Geometry check sheet. Reference: the model listing, model coordinates, mm. A direction names the side the tool comes from. Round coordinates to 2 decimals unless told otherwise and drop trailing zeros. Write each loop counter-clockwise with the first axis right and the second up, starting at its lowest first coordinate (ties: lowest second). Pieces come first, ordered by that corner, then holes. Notation, with made-up numbers: M 31.5,86.5 L 68.5,86.5 A20 ccw 68.5,120.5 Z; hole C 65,11 d4. An arc over 180 degrees is marked long. One line per item, written item: value. Start each with the question number.
1. Section check D-D (x = 57). Record the boundary of the cut face in (y, z), and give its area (3 significant figures).
2. Section check A-A (z = 3.25). Record the boundary of the cut face in (x, y), and give its area (3 significant figures).
3. Scan lines: probe 1 along Y at (x, z) = (1.5, -1.5); probe 2 along Y at (x, z) = (-9, 3); probe 3 along Y at (x, z) = (28.5, 4.75). Record each from-to range of solid material in increasing order. Write a range as [from, to].
4. Section check C-C (y = -9.5). Record the boundary of the cut face in (x, z), and give its area (3 significant figures).
5. Release check for a two-part mould opening along Y. For faces 1 (the flat face through (27, -3.84, 0)), 2 (the cylindrical face through (61.51, -5.044, -0.095)), 3 (the cylindrical face through (-5.43, -3.24, -0.1)), 4 (the flat face through (47.343, -17, 0)) record: pulls with the +Y half, pulls with the -Y half, needs draft (parallel to the pull), parting line crosses it, or undercut.
6. Access from +Z, -Z, +X, -X, +Y, -Y to the whole of each face (thin tool, end or side, straight path). Record for faces 5 (the flat face through (-7, 23, 0)), 6 (the flat face through (50, -16, 0)), 7 (the flat face through (19.84, 43, 0)), 8 (the flat face through (51, -20, 0)).
7. Depth check by flat-ended pin: P1, Ø8, axis at y = 10, z = 3.5, coming from the +X side; P2, Ø10, axis at y = 14.5, z = -2, coming from the -X side; P3, Ø5, axis at y = 5, z = 4, coming from the -X side; P4, Ø8, axis at x = 41, y = -11.5, coming from the -Z side. Enter the tip coordinate at first touch or a pass-through.
8. Section check B-B (x = 8). Record the boundary of the cut face in (y, z).
from build123d import *

# Parameters (mm, degrees)
F1_DEPTH = 30
F5_REACH = 130.7668048394
F6_DEPTH = 30
F8_R     = 2


# Not quite as in the source:
# - two fillets or chamfers of one size are made in one step


with BuildPart() as f1:
    # F0 (on Top) → F1 (new body, symmetric)
    with BuildSketch(Plane.XY):
        with BuildLine():
            Line((-2.159999702, 23), (-10.159999702, 23))
            Line((-10.159999702, 23), (-10.159999702, 41))
            Line((-10.159999702, 41), (19.840000298, 41))
            Line((19.840000298, 41), (19.840000298, 44.84))
            Line((19.840000298, 44.84), (-13.999999702, 44.84))
            Line((-13.999999702, 44.84), (-13.999999702, 19.16))
            Line((-13.999999702, 19.16), (-5.999999702, 19.16))
            Line((-5.999999702, 19.16), (-5.999999702, -3.84))
            Line((-5.999999702, -3.84), (64.5031457505, -3.84))
            Line((64.5031457505, -3.84), (52.6360389693, -15.7071067812))
            ThreePointArc((52.6360389693, -15.7071067812), (52.3116156205, -15.9238795325), (51.9289321881, -16))
            Line((51.9289321881, -16), (47.3431457505, -16))
            Line((47.3431457505, -16), (47.3431457505, -20))
            Line((47.3431457505, -20), (54, -20))
            Line((54, -20), (70, -4))
            Line((70, -4), (70, 0))
            Line((70, 0), (-2.159999702, 0))
            Line((-2.159999702, 0), (-2.159999702, 23))
        make_face()
    extrude(amount=F1_DEPTH, both=True)

    f5_end = Plane(origin=(0, -0.6162060448, 7.0432673219), x_dir=(0, 0.9961946981, 0.0871557427), z_dir=(0, -0.0871557427, 0.9961946981))
    # F1_face2 (on face) → F5 (cut, up to a plane its end follows)
    with BuildSketch(Plane(origin=(19.935386065, 10.6416249654, 30), x_dir=(1, 0, 0), z_dir=(0, 0, 1))):
        with BuildLine():
            Line((-22.095385767, -10.6416249654), (-22.095385767, 12.3583750346))
            Line((-22.095385767, 12.3583750346), (-30.095385767, 12.3583750346))
            Line((-30.095385767, 12.3583750346), (-30.095385767, 30.3583750346))
            Line((-30.095385767, 30.3583750346), (-0.095385767, 30.3583750346))
            Line((-0.095385767, 30.3583750346), (-0.095385767, 34.1983750346))
            Line((-0.095385767, 34.1983750346), (-33.935385767, 34.1983750346))
            Line((-33.935385767, 34.1983750346), (-33.935385767, 8.5183750346))
            Line((-33.935385767, 8.5183750346), (-25.935385767, 8.5183750346))
            Line((-25.935385767, 8.5183750346), (-25.935385767, -14.4816249654))
            Line((-25.935385767, -14.4816249654), (44.5677596855, -14.4816249654))
            Line((44.5677596855, -14.4816249654), (32.7006529043, -26.3487317465))
            ThreePointArc((32.7006529043, -26.3487317465), (32.3762295555, -26.5655044979), (31.9935461231, -26.6416249654))
            Line((31.9935461231, -26.6416249654), (27.4077596855, -26.6416249654))
            Line((27.4077596855, -26.6416249654), (27.4077596855, -30.6416249654))
            Line((27.4077596855, -30.6416249654), (34.064613935, -30.6416249654))
            Line((34.064613935, -30.6416249654), (50.064613935, -14.6416249654))
            Line((50.064613935, -14.6416249654), (50.064613935, -10.6416249654))
            Line((50.064613935, -10.6416249654), (-22.095385767, -10.6416249654))
        make_face()
    f5_long = extrude(amount=-F5_REACH, mode=Mode.PRIVATE)
    add(split(f5_long, bisect_by=f5_end, keep=Keep.TOP, mode=Mode.PRIVATE), mode=Mode.SUBTRACT)

    # F6 (cut, through all): a face of the model
    f6_faces = [f1.faces().sort_by_distance(p)[0] for p in [
        (-3.2211418013, 11.5, -30),
    ]]
    extrude(f6_faces, amount=-F6_DEPTH, mode=Mode.SUBTRACT)

    # F7: F1 across plane


with BuildPart() as f1_1:
    add(f1.part)
    add(f1.part.mirror(Plane.XY))

    # F8
    f8_edges = [f1_1.edges().sort_by_distance(p)[0] for p in [
        (70, 0, 0),
        (70, -4, 0),
        (54, -20, 0),
        (47.343146, -20, 0),
        (-2.16, 23, 0),
        (-14, 44.84, 0),
        (-14, 19.16, 0),
        (-6, 19.16, 0),
        (-6, -3.84, 0),
        (64.503146, -3.84, 0),
    ]]
    fillet(f8_edges, radius=F8_R)


solid = f1_1.part
Result sheet:
1. outline: M -17,-5.61 L -11.34,-6.1 L -11.34,6.1 L -17,5.61 Z; M -3.84,-6.76 L 0,-7.1 L 0,7.1 L -3.84,6.76 Z
1. area: 119 mm2
2. outline: M -14,21.16 A2 ccw -12,19.16 L -8,19.16 A2 cw -6,17.16 L -6,-1.84 A2 ccw -4,-3.84 L 59.67,-3.84 A2 cw 61.09,-7.25 L 52.64,-15.71 A1 cw 51.93,-16 L 47.34,-16 L 47.34,-18 A2 ccw 49.34,-20 L 53.17,-20 A2 ccw 54.59,-19.41 L 69.41,-4.59 A2 ccw 70,-3.17 L 70,-2 A2 ccw 68,0 L -2.16,0 L -2.16,21 A2 ccw -4.16,23 L -10.16,23 L -10.16,41 L 19.84,41 L 19.84,44.84 L -12,44.84 A2 ccw -14,42.84 Z
2. area: 714 mm2
3. probe 1: y = [-3.84, 0], [41, 44.84]
3. probe 2: y = [19.16, 23], [41, 44.84]
3. probe 3: y = [-3.84, 0]
4. outline: M 58.84,-6.27 L 64.5,-6.27 L 64.5,6.27 L 58.84,6.27 Z
4. area: 70.9 mm2
5. face 1: undercut
5. face 2: undercut
5. face 3: pulls with the -Y half
5. face 4: needs draft
6. face 5: +Z, -Z, +X
6. face 6: +Z, -Z, -X
6. face 7: +Z, -Z, +X, +Y
6. face 8: +Z, -Z, +X, -X, -Y
7. P1: stops at x = -2.16
7. P2: stops at x = -13.12
7. P3: stops at x = -6
7. P4: passes through
8. outline: M -3.84,-6.76 L 0,-7.1 L 0,7.1 L -3.84,6.76 Z; M 41,-10.68 L 44.84,-11.02 L 44.84,11.02 L 41,10.68 Z
